```python
from build123d import *

# Parameters (mm, degrees)
SKETCH_1_W          = 9
SKETCH_1_H          = 250
EXTRUDE_1_DEPTH     = 6.5
SKETCH_2_R          = 1.6
CUT_EXTRUDE_1_DEPTH = 126.249750499
SKETCH_3_R          = 3.25
CUT_EXTRUDE_2_DEPTH = 3
SKETCH_4_W          = 6.5
SKETCH_4_H          = 15
CUT_EXTRUDE_3_DEPTH = 10


with BuildPart() as part:
    # 草图1 → 凸台-拉伸1 (new body)
    with BuildSketch(Plane.XY):
        Rectangle(SKETCH_1_W, SKETCH_1_H)
    extrude(amount=EXTRUDE_1_DEPTH)

    # 草图2 → 切除-拉伸1 (cut, through all)
    with BuildSketch(Plane.XY.offset(6.5)):
        Circle(SKETCH_2_R)
        with Locations((0, 20)):
            Circle(SKETCH_2_R)
        with Locations((0, 40)):
            Circle(SKETCH_2_R)
        with Locations((0, 60)):
            Circle(SKETCH_2_R)
        with Locations((0, 80)):
            Circle(SKETCH_2_R)
        with Locations((0, -20)):
            Circle(SKETCH_2_R)
        with Locations((0, -40)):
            Circle(SKETCH_2_R)
        with Locations((0, -60)):
            Circle(SKETCH_2_R)
        with Locations((0, -80)):
            Circle(SKETCH_2_R)
    extrude(amount=-CUT_EXTRUDE_1_DEPTH, mode=Mode.SUBTRACT)

    # 草图3 → 切除-拉伸2 (cut)
    with BuildSketch(Plane.XY.offset(6.5)):
        with Locations((0, 80)):
            Circle(SKETCH_3_R)
        with Locations((0, 60)):
            Circle(SKETCH_3_R)
        with Locations((0, 40)):
            Circle(SKETCH_3_R)
        with Locations((0, 20)):
            Circle(SKETCH_3_R)
        Circle(SKETCH_3_R)
        with Locations((0, -20)):
            Circle(SKETCH_3_R)
        with Locations((0, -40)):
            Circle(SKETCH_3_R)
        with Locations((0, -60)):
            Circle(SKETCH_3_R)
        with Locations((0, -80)):
            Circle(SKETCH_3_R)
    extrude(amount=-CUT_EXTRUDE_2_DEPTH, mode=Mode.SUBTRACT)

    # 草图4 → 切除-拉伸3 (cut)
    with BuildSketch(Plane.ZY.offset(4.5)):
        with Locations((3.25, -117.5)):
            Rectangle(SKETCH_4_W, SKETCH_4_H)
    extrude(amount=-CUT_EXTRUDE_3_DEPTH, mode=Mode.SUBTRACT)


solid = part.part
```
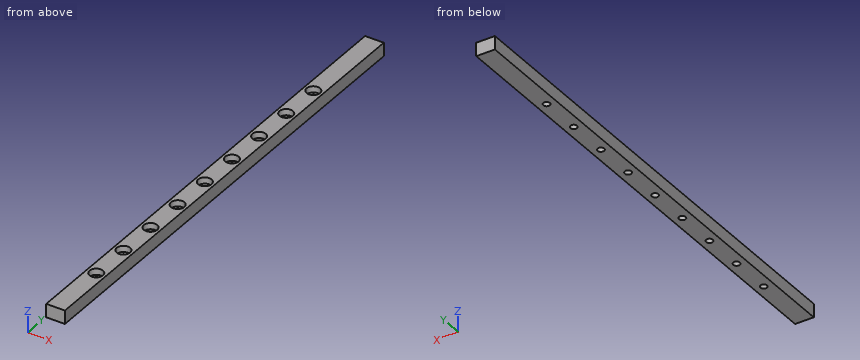
CAD build for the part. Positions are in the model's coordinates, mm. Coordinates: 2 decimals unless noted, no trailing zeros.
(1) Saw through at A-A, the plane z = 1. Count the separate pieces of the cut face and the enclosed holes in it, and give its area (3 significant figures).
Solution:
separate pieces: 1
enclosed holes: 9
area: 2,040 mm2
(2) Drill centre lines: L1, parallel to X at y = -80, z = 0.9; L2, parallel to X at y = -1, z = 1.75; L3, parallel to Z at x = -0.5, y = 37. Where is each one in solid material? Low to high.
Solution:
L1: x = -4.5 to -1.6, 1.6 to 4.5
L2: x = -4.5 to -1.25, 1.25 to 4.5
L3: z = 0 to 3.5
(3) Pin check, flat tip, straight feed: pin 1 Ø4 at (x, y) = (0, 40) entering from +Z. Stop position of the tip, or through.
Solution:
pin 1: stops at z = 3.5
